```python
from build123d import *

# Parameters (mm, degrees)
F0_R      = 9
F1_DEPTH  = 24.5
F2_R      = 9
F3_DEPTH  = 14
F4_R      = 30
F5_DEPTH  = 8
F6_SIZE   = 1.5
F7_R      = 28.5
F8_DEPTH  = 32
F9_SIZE   = 1.5
F10_R     = 16
F11_DEPTH = 89.001
F12_R     = 64.5
F12_R_2   = 16
F13_DEPTH = 30
F14_R     = 12
F14_R_2   = 6.35
F15_DEPTH = 2
F16_DEPTH = 9


with BuildPart() as f1:
    # F0 (on Front) → F1 (new body, symmetric)
    with BuildSketch(Plane.XZ):
        with BuildLine():
            Line((-60, -70), (60, -70))
            ThreePointArc((60, -70), (67.0710678119, -67.0710678119), (70, -60))
            Line((70, -60), (70, 60))
            ThreePointArc((70, 60), (67.0710678119, 67.0710678119), (60, 70))
            Line((60, 70), (-60, 70))
            ThreePointArc((-60, 70), (-67.0710678119, 67.0710678119), (-70, 60))
            Line((-70, 60), (-70, -60))
            ThreePointArc((-70, -60), (-67.0710678119, -67.0710678119), (-60, -70))
        make_face()
        with Locations((-55, -55)):
            Circle(F0_R, mode=Mode.SUBTRACT)
        with Locations((55, -55)):
            Circle(F0_R, mode=Mode.SUBTRACT)
        with Locations((-55, 55)):
            Circle(F0_R, mode=Mode.SUBTRACT)
        with Locations((55, 55)):
            Circle(F0_R, mode=Mode.SUBTRACT)
    extrude(amount=F1_DEPTH, both=True)

    # F2 (on face) → F3 (cut)
    with BuildSketch(Plane.XZ.offset(24.5)):
        with BuildLine():
            Line((30, -50), (30, -70))
            Line((30, -70), (60, -70))
            ThreePointArc((60, -70), (67.0710678119, -67.0710678119), (70, -60))
            Line((70, -60), (70, -30))
            Line((70, -30), (50, -30))
            ThreePointArc((50, -30), (35.8578643763, -35.8578643763), (30, -50))
        make_face()
        with Locations((55, -55)):
            Circle(F2_R, mode=Mode.SUBTRACT)
        with BuildLine():
            Line((60, 70), (30, 70))
            Line((30, 70), (30, 50))
            ThreePointArc((30, 50), (35.8578643763, 35.8578643763), (50, 30))
            Line((50, 30), (70, 30))
            Line((70, 30), (70, 60))
            ThreePointArc((70, 60), (67.0710678119, 67.0710678119), (60, 70))
        make_face()
        with Locations((55, 55)):
            Circle(F2_R, mode=Mode.SUBTRACT)
        with BuildLine():
            Line((-70, 60), (-70, 30))
            Line((-70, 30), (-50, 30))
            ThreePointArc((-50, 30), (-35.8578643763, 35.8578643763), (-30, 50))
            Line((-30, 50), (-30, 70))
            Line((-30, 70), (-60, 70))
            ThreePointArc((-60, 70), (-67.0710678119, 67.0710678119), (-70, 60))
        make_face()
        with Locations((-55, 55)):
            Circle(F2_R, mode=Mode.SUBTRACT)
        with BuildLine():
            Line((-50, -30), (-70, -30))
            Line((-70, -30), (-70, -60))
            ThreePointArc((-70, -60), (-67.0710678119, -67.0710678119), (-60, -70))
            Line((-60, -70), (-30, -70))
            Line((-30, -70), (-30, -50))
            ThreePointArc((-30, -50), (-35.8578643763, -35.8578643763), (-50, -30))
        make_face()
        with Locations((-55, -55)):
            Circle(F2_R, mode=Mode.SUBTRACT)
    extrude(amount=-F3_DEPTH, mode=Mode.SUBTRACT)

    # F4 (on face) → F5 (join)
    with BuildSketch(Plane.XZ.offset(24.5)):
        Circle(F4_R)
    extrude(amount=F5_DEPTH)

    # F6
    f6_edges = [f1.edges().sort_by_distance(p)[0] for p in [
        (-30, -32.5, 0),
    ]]
    chamfer(f6_edges, length=F6_SIZE)

    # F7 (on face) → F8 (join)
    with BuildSketch(Plane.XZ.offset(32.5)):
        Circle(F7_R)
    extrude(amount=F8_DEPTH)

    # F9
    f9_edges = [f1.edges().sort_by_distance(p)[0] for p in [
        (-28.5, -64.5, 0),
    ]]
    chamfer(f9_edges, length=F9_SIZE)

    # F10 (on face) → F11 (cut, through all)
    with BuildSketch(Plane.XZ.offset(64.5)):
        Circle(F10_R)
    extrude(amount=-F11_DEPTH, mode=Mode.SUBTRACT)

    # F12 (on face) → F13 (cut)
    with BuildSketch(Plane(origin=(0, 24.5, 0), x_dir=(-1, 0, 0), z_dir=(0, 1, 0))):
        Circle(F12_R)
        Circle(F12_R_2, mode=Mode.SUBTRACT)
    extrude(amount=-F13_DEPTH, mode=Mode.SUBTRACT)

    # F14 (on face) → F15 (cut)
    with BuildSketch(Plane.YZ.offset(70)):
        with Locations((8.5, 7.547759451)):
            Circle(F14_R)
        with Locations((8.5, 7.547759451)):
            Circle(F14_R_2, mode=Mode.SUBTRACT)
    extrude(amount=-F15_DEPTH, mode=Mode.SUBTRACT)

    # F16 (cut): a face of the model
    f16_faces = [f1.faces().sort_by_distance(p)[0] for p in [
        (70, 8.5, 7.547759451),
    ]]
    extrude(f16_faces, amount=-F16_DEPTH, mode=Mode.SUBTRACT)


solid = f1.part
```
Input: part model. Units: mm. Frame: model coordinates. A direction names the side the tool comes from. Coordinates: 2 decimals unless noted, no trailing zeros. Order: outer loops, then holes, each group sorted by start corner. A loop starts at its lowest first (then second) coordinate and runs counter-clockwise, first axis right, second up. Notation, with made-up numbers: (-5.75, 75) - (-1.75, 75) arc R22 cw to (-1.75, 93) - close; hole circle Ø8 at (31.5, -3.75). An arc over 180 degrees is marked (long way). Put each result on its own line as item: value.
1. Cut plane C-C on y = 8.5. Return the cut outline in (x, z).
Report:
outline: (-70, -60) arc R10 ccw to (-60, -70) - (60, -70) arc R10 ccw to (70, -60) - (70, -4.45) - (68, -4.45) - (68, 1.2) - (64.49, 1.2) arc R64.5 cw (long way) to (62.98, 13.9) - (68, 13.9) - (68, 19.55) - (70, 19.55) - (70, 60) arc R10 ccw to (60, 70) - (-60, 70) arc R10 ccw to (-70, 60) - close; hole circle Ø18 at (-55, -55); hole circle Ø18 at (-55, 55); hole circle Ø18 at (55, -55); hole circle Ø18 at (55, 55)
2. Draft query along X for faces 5 (the face through (-13, -5.5, -13)), 6 (the face through (70, -0.34, -0.84)), 7 (the face through (59.84, 7.25, 62.59)), 8 (the face through (12, -64.5, -12)). Return one class per face: pulls with the +X half, pulls with the -X half, needs draft (parallel to the pull), parting line crosses it, or undercut.
Report:
face 5: undercut
face 6: pulls with the +X half
face 7: undercut
face 8: needs draft
3. Cut plane A-A on z = -55. Return the cut outline in (x, y).
Report:
outline: (-70, -10.5) - (-64, -10.5) - (-64, 24.5) - (-70, 24.5) - close; (-46, -10.5) - (-30, -10.5) - (-30, -24.5) - (30, -24.5) - (30, -10.5) - (46, -10.5) - (46, 24.5) - (33.69, 24.5) - (33.69, -5.5) - (-33.69, -5.5) - (-33.69, 24.5) - (-46, 24.5) - close; (64, -10.5) - (70, -10.5) - (70, 24.5) - (64, 24.5) - close
4. Line query: line 1 along X through (y, z) = (9, 58.5); line 2 along X through (y, z) = (-2.5, 53); line 3 along Y through (x, z) = (35.5, 48.5). Output: solid intervals per line, ascending.
Report:
line 1: x = -70 to -63.29, -46.71 to -27.17, 27.17 to 46.71, 63.29 to 70
line 2: x = -70 to -63.77, -46.23 to -36.76, 36.76 to 46.23, 63.77 to 70
line 3: y = -10.5 to -5.5
5. Cut plane D-D on x = -41. Return the cut outline in (y, z).
Report:
outline: (-24.5, -32.14) - (-10.5, -32.14) - (-10.5, -70) - (24.5, -70) - (24.5, -49.79) - (-5.5, -49.79) - (-5.5, 49.79) - (24.5, 49.79) - (24.5, 70) - (-10.5, 70) - (-10.5, 32.14) - (-24.5, 32.14) - close
6. Contact query for flat-ended pins moving along their axis: pin 1 Ø12 at (x, z) = (-41, -24.5) entering from -Y; pin 2 Ø15.5 at (y, z) = (-17.5, -62) entering from +X; pin 3 Ø1.5 at (y, z) = (-18.5, -34) entering from -X; pin 4 Ø4 at (y, z) = (-20, 56) entering from -X. Output: stop coordinate, or through.
Report:
pin 1: stops at y = -24.5
pin 2: stops at x = 70
pin 3: stops at x = -39.07
pin 4: stops at x = -30
7. Reachability of faces 1 (the face through (-30, -18, 60)), 2 (the face through (69.014, 19.585, 2.952)), 3 (the face through (60, -18, 30)), 4 (the face through (60, -18, -30)) from +Z, -Z, +X, -X, +Y, -Y: full face, straight path, thin tool, end or side. Return the list, or none.
Report:
face 1: +Z, -X, -Y
face 2: +X
face 3: +Z, +X, -Y
face 4: -Z, +X, -Y
8. Cut plane B-B on x = 52. Return the cut outline in (y, z).
Report:
outline: (-24.5, -30) - (-10.5, -30) - (-10.5, -46.51) - (24.5, -46.51) - (24.5, -38.16) - (-5.5, -38.16) - (-5.5, 38.16) - (24.5, 38.16) - (24.5, 46.51) - (-10.5, 46.51) - (-10.5, 30) - (-24.5, 30) - close; (-10.5, -70) - (24.5, -70) - (24.5, -63.49) - (-10.5, -63.49) - close; (-10.5, 63.49) - (24.5, 63.49) - (24.5, 70) - (-10.5, 70) - close
